from build123d import *

# Parameters (mm, degrees)
CROQUIS1_R              = 65
SALIENTE_EXTRUIR2_DEPTH = 12


with BuildPart() as part:
    # Croquis1 → Saliente-Extruir2 (new body)
    with BuildSketch(Plane(origin=(0, 0, 0), x_dir=(1, 0, 0), z_dir=(0, 1, 0))):
        with BuildLine():
            Line((57, 0), (57, 104.820295074))
            ThreePointArc((57, 104.820295074), (180, 227.820295074), (303, 104.820295074))
            Line((303, 104.820295074), (303, 0))
            Line((303, 0), (295.121320344, 0))
            ThreePointArc((295.121320344, 0), (293, 0), (293, -2.121320344))
            Line((293, -2.121320344), (293, -12))
            Line((293, -12), (253, -12))
            Line((253, -12), (253, -2.121320344))
            ThreePointArc((253, -2.121320344), (253, 0), (250.878679656, 0))
            Line((250.878679656, 0), (233.121320344, 0))
            ThreePointArc((233.121320344, 0), (231, 0), (231, -2.121320344))
            Line((231, -2.121320344), (231, -12))
            Line((231, -12), (191, -12))
            Line((191, -12), (191, -2.121320344))
            ThreePointArc((191, -2.121320344), (191, 0), (188.878679656, 0))
            Line((188.878679656, 0), (171.121320344, 0))
            ThreePointArc((171.121320344, 0), (169, 0), (169, -2.121320344))
            Line((169, -2.121320344), (169, -12))
            Line((169, -12), (129, -12))
            Line((129, -12), (129, -2.121320344))
            ThreePointArc((129, -2.121320344), (129, 0), (126.878679656, 0))
            Line((126.878679656, 0), (109.121320344, 0))
            ThreePointArc((109.121320344, 0), (107, 0), (107, -2.121320344))
            Line((107, -2.121320344), (107, -12))
            Line((107, -12), (67, -12))
            Line((67, -12), (67, -2.121320344))
            ThreePointArc((67, -2.121320344), (67, 0), (64.878679656, 0))
            Line((64.878679656, 0), (57, 0))
        make_face()
        with Locations(Location((180, 104.820295074, 0), (0, 0, 270))):
            Circle(CROQUIS1_R, mode=Mode.SUBTRACT)
    extrude(amount=SALIENTE_EXTRUIR2_DEPTH)


solid = part.part
Check sheet for the modelled part. Datum: model origin and axes. Units: mm. A direction names the side the tool comes from. Give positions to 0.01 mm unless a question says otherwise; leave off trailing zeros. Loops run counter-clockwise (first coordinate to the right, second up) from the corner with the lowest first, then second, coordinate; pieces in that order, holes last. Notation, with made-up numbers: M 46.25,12 L 82.25,12 A20 ccw 82.25,19 Z; hole C 4.25,60.25 d11. An arc over 180 degrees is marked long. Use a Markdown table: item, result. Add a question column.
Q1. Mould release check, pull along X, two halves, no side actions. Record for faces 6 (the flat face through (169, 6, 7)), 7 (the flat face through (182, 12, -30)), 8 (the flat face through (57, 6, -52)): pulls with the +X half, pulls with the -X half, needs draft (parallel to the pull), parting line crosses it, or undercut.
Q2. Scan lines: line 1 along Z through (x, y) = (200.5, 6); line 2 along X through (y, z) = (1, -59); line 3 along Z through (x, y) = (196, 1.5). Record each from-to range of solid material in increasing order. Write a range as [from, to].
Q3. Tool access check on faces 1 (the flat face through (61, 6, 0)), 2 (the flat face through (129, 6, 7)), 3 (the flat face through (273, 6, 12)), 4 (the flat face through (293, 6, 7)), 5 (the flat face through (182, 0, -30)). Record the directions out of +Z, -Z, +X, -X, +Y, -Y that give a thin tool (end or side, any length) a straight path to the whole face; none if there is none.
Q4. Go/stop test with flat-tipped pins: pin 1 (1 mm diameter, centred on x = 251, y = 8.5, fed in from -Z); pin 2 (5 mm diameter, centred on y = 5, z = 9, fed in from +X); pin 3 (6 mm diameter, centred on x = 178.5, y = 8, fed in from +Z). Record where each tip stops, or that it passes through.
Q5. Sectioned sample at A-A, the plane x = 180. Record the cut outline in (y, z), then the cut area to 3 significant figures.
Q6. Sectioned sample at D-D, the plane z = -194.5. Record the cut outline in (x, y).
Q7. Sectioned sample at C-C, the plane z = -162.5. Record the cut outline in (x, y).
Verdict:
| question | item | result |
|---|---|---|
| 1 | face 6 | undercut |
| 1 | face 7 | needs draft |
| 1 | face 8 | pulls with the -X half |
| 2 | line 1 | [-226.1, -166.5], [-43.14, 12] |
| 2 | line 2 | [57, 133.9], [226.1, 303] |
| 2 | line 3 | [-226.78, -167.82], [-41.82, 12] |
| 3 | face 1 | +Z, -X, +Y, -Y |
| 3 | face 2 | +Z, +Y, -Y |
| 3 | face 3 | +Z, +X, -X, +Y, -Y |
| 3 | face 4 | +Z, +X, +Y, -Y |
| 3 | face 5 | +Z, -Z, +X, -X, -Y |
| 4 | pin 1 | z = -205.61 |
| 4 | pin 2 | x = 293 |
| 4 | pin 3 | z = 0 |
| 5 | outline | M 0,-227.82 L 12,-227.82 L 12,-169.82 L 0,-169.82 Z; M 0,-39.82 L 12,-39.82 L 12,0 L 0,0 Z |
| 5 | area | 1,170 mm^2 |
| 6 | outline | M 95.82,0 L 264.18,0 L 264.18,12 L 95.82,12 Z |
| 7 | outline | M 71.36,0 L 150.03,0 L 150.03,12 L 71.36,12 Z; M 209.97,0 L 288.64,0 L 288.64,12 L 209.97,12 Z |
